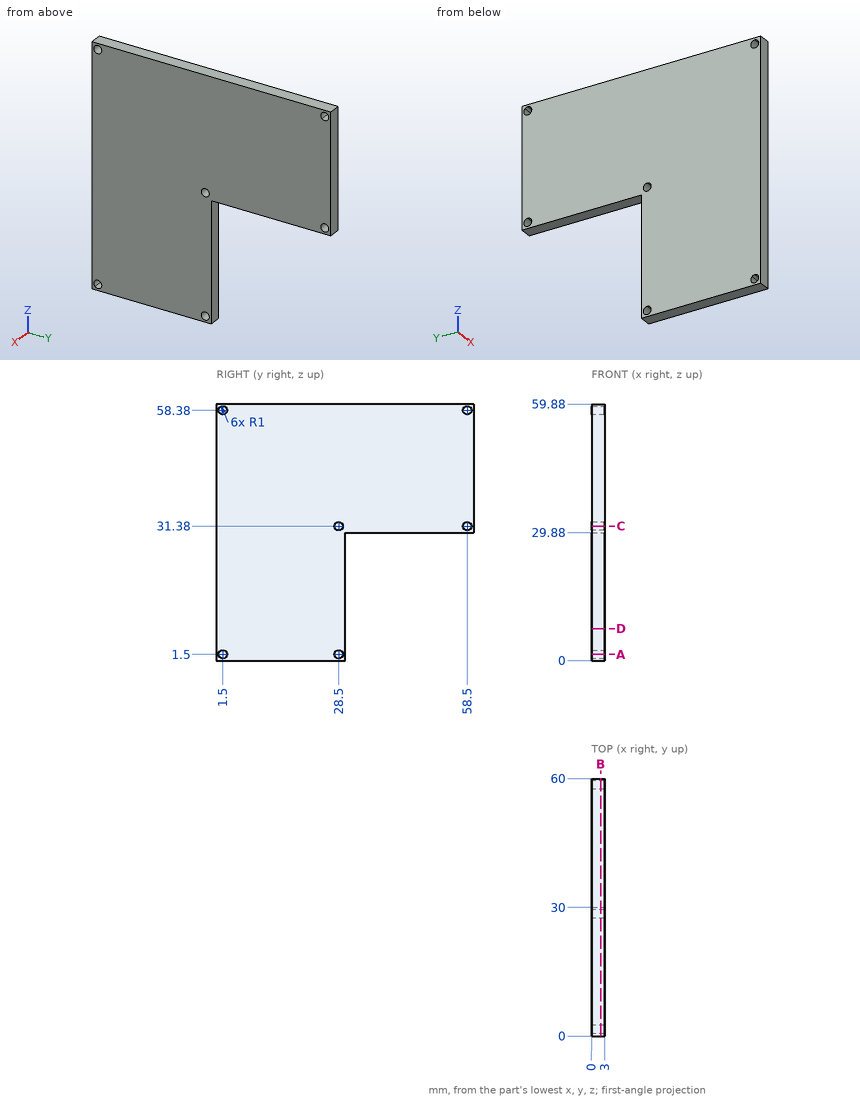
The figure shows three views and two pictorial views of one solid part (mm, origin at its lowest corner). Answer the questions. Give positions to 0.01 mm unless a question says otherwise; leave off trailing zeros. Order: outer loops, then holes, each group sorted by start corner. A loop starts at its lowest first (then second) coordinate and runs counter-clockwise, first axis right, second up. Notation, with made-up numbers: (77.25, 66) -> (129.25, 66) arc R16 ccw to (129.25, 91) -> close; hole circle Ø1 at (32, -29). An arc over 180 degrees is marked (long way). Answer as a JSON object with one key per item and string values. Group by question number.
Item 1: The part is cut by section D-D on z = 7.5. Write down the section's boundary in (x, y).
Item 2: A flat-ended cylindrical pin translates along its axis: pin 1 (0.9 mm diameter, centred on x = 1.5, z = 12, fed in from +Y). Find the tip coordinate at first contact, or state that the pin passes through.
Item 3: The part is cut by section B-B on x = 2.1. Write down the section's boundary in (y, z), and give its area (3 significant figures).
Item 4: The part is cut by section C-C on z = 31.38. Write down the section's boundary in (x, y), and give its area (3 significant figures).
Item 5: The part is cut by section A-A on z = 1.5. Write down the section's boundary in (x, y).
Item 6: Consider L1, parallel to Y at x = 2.05, z = 30.5; L2, parallel to Y at x = 1.6, z = 3.5; L3, parallel to Z at x = 0.6, y = 50.5. Determine where each line is inside the solid, lowest interval first. Write a range as from..to.
Result set:
{
 "1": {"outline": "(0, 0) -> (3, 0) -> (3, 30) -> (0, 30) -> close"},
 "2": {"pin 1": "y = 30"},
 "3": {"outline": "(0, 0) -> (30, 0) -> (30, 29.88) -> (60, 29.88) -> (60, 59.88) -> (0, 59.88) -> close; hole circle Ø2 at (1.5, 1.5); hole circle Ø2 at (1.5, 58.38); hole circle Ø2 at (28.5, 1.5); hole circle Ø2 at (28.5, 31.38); hole circle Ø2 at (58.5, 31.38); hole circle Ø2 at (58.5, 58.38)", "area": "2,680 mm²"},
 "4": {"outline": "(0, 0) -> (3, 0) -> (3, 27.5) -> (0, 27.5) -> close; (0, 29.5) -> (3, 29.5) -> (3, 57.5) -> (0, 57.5) -> close; (0, 59.5) -> (3, 59.5) -> (3, 60) -> (0, 60) -> close", "area": "168 mm²"},
 "5": {"outline": "(0, 0) -> (3, 0) -> (3, 0.5) -> (0, 0.5) -> close; (0, 2.5) -> (3, 2.5) -> (3, 27.5) -> (0, 27.5) -> close; (0, 29.5) -> (3, 29.5) -> (3, 30) -> (0, 30) -> close"},
 "6": {"L1": "0..28.03, 28.97..58.03, 58.97..60", "L2": "0..30", "L3": "29.88..59.88"}
}
